For this review, use the dimensioned drawing (mm, ordinates from the lowest corner) and the shaded views. Round coordinates to 2 decimals unless told otherwise and drop trailing zeros. Write each loop counter-clockwise with the first axis right and the second up, starting at its lowest first coordinate (ties: lowest second). Pieces come first, ordered by that corner, then holes. Notation, with made-up numbers: (87.25, 76.25) - (116.25, 76.25) arc R19 ccw to (116.25, 107.25) - close; hole circle Ø11 at (63, 14.5). An arc over 180 degrees is marked (long way). Return JSON: item names as keys, results as strings.
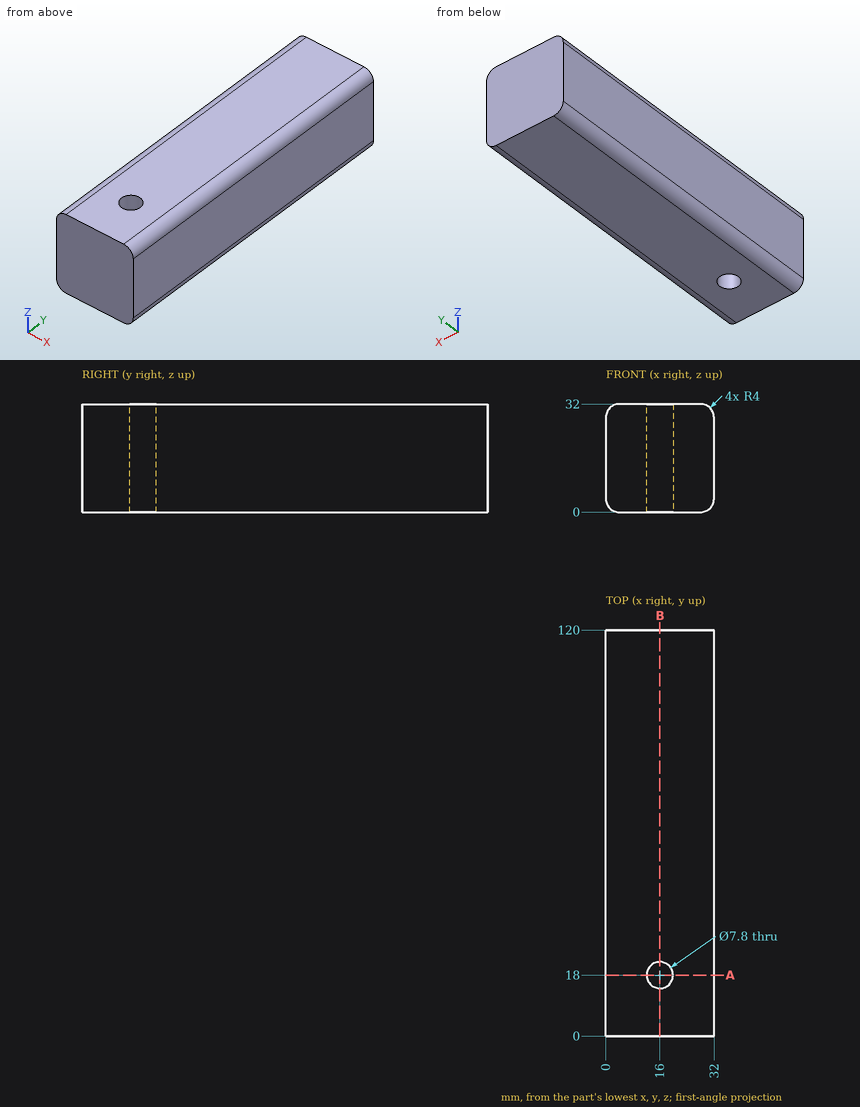
(1) Clearance check with a flat-ended pin moving along its axis: pin 1 Ø2 at (y, z) = (95, 15.5) entering from -X. State where the tip first meets the part, or that it passes through.
Filled in:
{"pin 1": "stops at x = 0"}
(2) Add section B-B (x = 16). Write out the cut boundary in (y, z), plus the area to 3 significant figures.
Filled in:
{"outline": "(0, 0) - (14.1, 0) - (14.1, 32) - (0, 32) - close; (21.9, 0) - (120, 0) - (120, 32) - (21.9, 32) - close", "area": "3,590 mm2"}
(3) Wall thickness on line 1 (Y direction, x = 16, z = 11); line 2 (Y direction, x = 13.5, z = 17); line 3 (Z direction, x = 3.5, y = 42): over which ranges is each line inside the solid? List them lowest first.
Filled in:
{"line 1": "y = 0 to 14.1, 21.9 to 120", "line 2": "y = 0 to 15.01, 20.99 to 120", "line 3": "z = 0.03 to 31.97"}
(4) Add section A-A (y = 18). Write out the cut boundary in (x, z), plus the area to 3 significant figures.
Filled in:
{"outline": "(0, 4) arc R4 ccw to (4, 0) - (12.1, 0) - (12.1, 32) - (4, 32) arc R4 ccw to (0, 28) - close; (19.9, 0) - (28, 0) arc R4 ccw to (32, 4) - (32, 28) arc R4 ccw to (28, 32) - (19.9, 32) - close", "area": "761 mm2"}
